Part model, mm, in its own coordinate system. Face numbers are marked on the shaded views. A direction names the side the tool comes from. Coordinates: 2 decimals unless noted, no trailing zeros. Write each loop counter-clockwise with the first axis right and the second up, starting at its lowest first coordinate (ties: lowest second). Pieces come first, ordered by that corner, then holes. Notation, with made-up numbers: M -21.75,51.5 L 36.25,51.5 A15 ccw 36.25,65.5 Z; hole C 20,26 d6. An arc over 180 degrees is marked long. Use a Markdown table: item, result. Add a question column.
Q1. Slice it at B-B on x = 215. Write the cut outline in (y, z).
Q2. Slice it at A-A on x = 252. Write the cut outline in (y, z).
Q3. Slice it at C-C on y = 0. Write the cut outline in (x, z), then the cut area to 3 significant figures.
Q4. Mould opens along Z. For the marked faces 6, 7, 8 and 9 say: released by +Z, released by -Z, zero draft, split by the parting line, or undercut.
Q5. Slice it at D-D on z = -40. Write the cut outline in (x, y).
Q6. Tool access for the marked faces 1, 2, 3, 4 and 5: list every direction of +Z, -Z, +X, -X, +Y, -Y with a clear straight run to the whole face (end or side of a thin tool).
Q7. Wall check: L1, parallel to Z at x = 243, y = -25; L2, parallel to Z at x = 260, y = -39.5; L3, parallel to Z at x = 51, y = 19. Give the ranges that are in metal, low to high. Write a range as from..to.
Q8. Pin check, flat tips, straight feed: pin 1 Ø12 at (x, z) = (91.5, 1) entering from +Y; pin 2 Ø6 at (y, z) = (22, 115) entering from -X; pin 3 Ø3 at (y, z) = (55.5, -21) entering from -X; pin 4 Ø10 at (x, y) = (230, -27) entering from -Z. Stop position of each tip, or through.
from build123d import *

# Parameters (mm, degrees)
BOSS_EXTRUDE1_DEPTH = 7.5
SKETCH3_W           = 100
SKETCH3_H           = 130
BOSS_EXTRUDE2_DEPTH = 150
SKETCH4_R           = 30
BOSS_EXTRUDE3_DEPTH = 100
SKETCH5_R           = 50
BOSS_EXTRUDE4_DEPTH = 50
SKETCH6_R           = 25
BOSS_EXTRUDE5_DEPTH = 100
SKETCH7_R           = 75
BOSS_EXTRUDE6_DEPTH = 8


with BuildPart() as part:
    # Sketch1 → Boss-Extrude1 (new body, symmetric)
    with BuildSketch(Plane.XY):
        with BuildLine():
            Line((0, 40), (140, 40))
            Line((140, 40), (140, -40))
            Line((140, -40), (0, -40))
            ThreePointArc((0, -40), (-40, 0), (0, 40))
        make_face()
    extrude(amount=BOSS_EXTRUDE1_DEPTH, both=True)

    # Sketch3 → Boss-Extrude2 (add)
    with BuildSketch(Plane(origin=(140, 0, 0), x_dir=(0, 0, -1), z_dir=(1, 0, 0))):
        Rectangle(SKETCH3_W, SKETCH3_H)
    extrude(amount=BOSS_EXTRUDE2_DEPTH)

    # Sketch4 → Boss-Extrude3 (add)
    with BuildSketch(Plane(origin=(0, 0, -50), x_dir=(-1, 0, 0), z_dir=(0, 0, -1))):
        with Locations((-215, 0)):
            Circle(SKETCH4_R)
    extrude(amount=BOSS_EXTRUDE3_DEPTH)

    # Sketch5 → Boss-Extrude4 (add)
    with BuildSketch(Plane.XY.offset(50)):
        with Locations((215, 0)):
            Circle(SKETCH5_R)
    extrude(amount=BOSS_EXTRUDE4_DEPTH)

    # Sketch6 → Boss-Extrude5 (add)
    with BuildSketch(Plane.XY.offset(100)):
        with Locations((215, 0)):
            Circle(SKETCH6_R)
    extrude(amount=BOSS_EXTRUDE5_DEPTH)

    # Sketch7 → Boss-Extrude6 (add)
    with BuildSketch(Plane.XY.offset(200)):
        with Locations((215, 0)):
            Circle(SKETCH7_R)
    extrude(amount=BOSS_EXTRUDE6_DEPTH)


solid = part.part
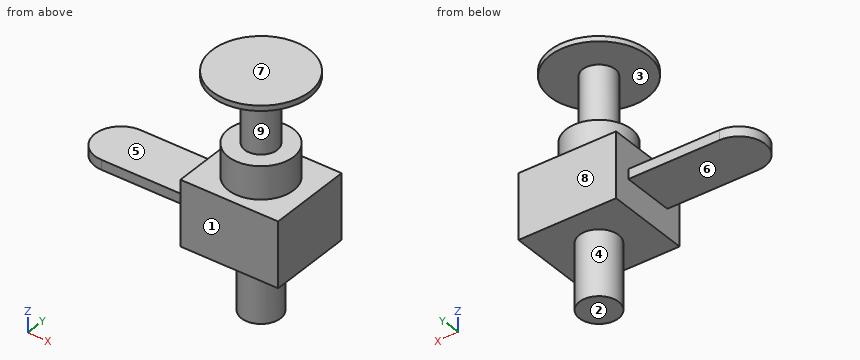
Recorded:
| question | item | result |
|---|---|---|
| 1 | outline | M -75,200 L -25,200 L -25,100 L -50,100 L -50,50 L -65,50 L -65,-50 L -30,-50 L -30,-150 L 30,-150 L 30,-50 L 65,-50 L 65,50 L 50,50 L 50,100 L 25,100 L 25,200 L 75,200 L 75,208 L -75,208 Z |
| 2 | outline | M -65.24,200 L 65.24,200 L 65.24,208 L -65.24,208 Z; M -65,-50 L 65,-50 L 65,50 L 33.63,50 L 33.63,100 L -33.63,100 L -33.63,50 L -65,50 Z |
| 3 | outline | M -40,-7.5 L 140,-7.5 L 140,-50 L 185,-50 L 185,-150 L 245,-150 L 245,-50 L 290,-50 L 290,50 L 265,50 L 265,100 L 240,100 L 240,200 L 290,200 L 290,208 L 140,208 L 140,200 L 190,200 L 190,100 L 165,100 L 165,50 L 140,50 L 140,7.5 L -40,7.5 Z |
| 3 | area | 34,900 mm² |
| 4 | face 6 | released by -Z |
| 4 | face 7 | released by +Z |
| 4 | face 8 | zero draft |
| 4 | face 9 | undercut |
| 5 | outline | M 140,-65 L 290,-65 L 290,65 L 140,65 Z |
| 6 | face 1 | -Z, +X, -X, -Y |
| 6 | face 2 | -Z, +X, -X, +Y, -Y |
| 6 | face 3 | none |
| 6 | face 4 | -Z |
| 6 | face 5 | +Z, -X, +Y, -Y |
| 7 | L1 | -50..100, 200..208 |
| 7 | L2 | -50..50, 200..208 |
| 7 | L3 | -7.5..7.5 |
| 8 | pin 1 | y = 40 |
| 8 | pin 2 | x = 198.75 |
| 8 | pin 3 | x = 140 |
| 8 | pin 4 | z = -150 |
